The model under review builds one solid part; all positions refer to its coordinate system, in mm. Face numbers are marked on the shaded views. Round coordinates to 2 decimals unless told otherwise and drop trailing zeros. Order: outer loops, then holes, each group sorted by start corner. A loop starts at its lowest first (then second) coordinate and runs counter-clockwise, first axis right, second up.
Autodesk Inventor part; units mm, degrees
ref_plane "YZ Plane" through (0, 0, 0) normal (1, 0, 0) x (0, 1, 0)
ref_plane "XZ Plane" through (0, 0, 0) normal (0, 1, 0) x (-1, 0, 0)
ref_plane "XY Plane" through (0, 0, 0) normal (0, 0, 1) x (1, 0, 0)
sketch "Эскиз1" plane through (0, 0, 0) normal (0, 1, 0) x (-1, 0, 0)
  line L0 (0, 0) -> (2.52, 0)
  line L1 (2.52, 0) -> (2.52, -2.52)
  line L2 (2.52, -2.52) -> (0, -2.52)
  line L3 (0, -2.52) -> (0, 0)
  dimension "d1" = 2.52
  dimension "d2" = 2.52
extrude "Выдавливание1" add sketch "Эскиз1" along normal blind 8
sketch "Эскиз2" plane through (0, 8, 0) normal (0, 1, 0) x (1, 0, 0)
  line L0 (-2.52, 2.52) -> (-2.52, 0) construction
  line L1 (0, 0) -> (0, 2.52) construction
  line L2 (-2.52, 0) -> (0, 2.52) construction
  circle A0 centre (-1.26, 1.26) radius 0.5
  dimension "d22" = 1
extrude "Выдавливание2" add sketch "Эскиз2" along normal blind 3.5
chamfer "Фаска3" distance 0.5 angle 45 1 edges at (-1.76, 11.5, -1.26)
sketch "Эскиз3" plane through (0, 0, 0) normal (0, -1, 0) x (1, 0, 0)
  line L0 (0, 0) -> (0, -2.52) construction
  line L1 (0, -2.52) -> (-2.52, -2.52) construction
  line L2 (0, 0) -> (-2.52, -2.52) construction
  line L3 (-1.81, -0.71) -> (-0.71, -0.71)
  line L4 (-0.71, -0.71) -> (-0.71, -1.81)
  line L5 (-0.71, -1.81) -> (-1.81, -1.81)
  line L6 (-1.81, -1.81) -> (-1.81, -0.71)
  line L7 (-1.81, -0.71) -> (-0.71, -1.81) construction
  line L8 (-0.71, -0.71) -> (-1.81, -1.81) construction
  point P0 (-1.26, -1.26)
  dimension "d15" = 1.1
  dimension "d16" = 1.1
extrude "Выдавливание3" cut sketch "Эскиз3" against normal blind 6
pattern_linear "Прямоуг.массив1" count 6 spacing 2.52 along (0, 0, 1) of "Выдавливание1", "Выдавливание2", "Выдавливание3", "Фаска3"
properties part number "Гребенка 20 МАМА"
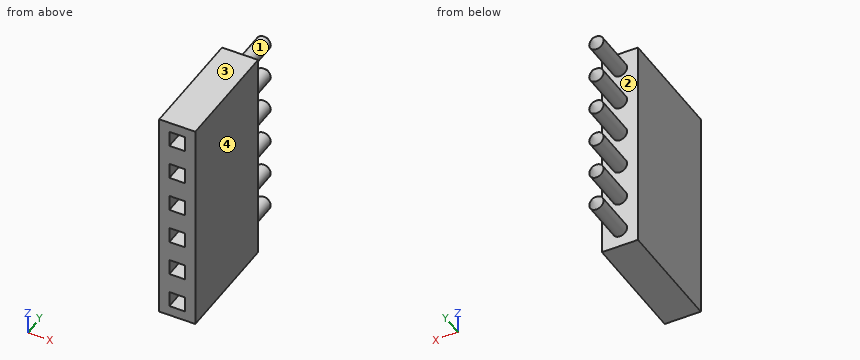
(1) We need section D-D (z = 7.75). Give the boundary of the cut face in (x, y), and give its area (3 significant figures).
(2) To check wall thickness, follow L1, parallel to X at y = 5.5, z = 8.5; L2, parallel to Z at x = -1, y = 8.5; L3, parallel to Y at x = -1, z = 5. State the ranges of each line that lie inside material, in increasing order.
(3) Clearance check with a flat-ended pin moving along its axis: P1, Ø2, axis at y = 9.5, z = 1, coming from the +X side. State where the tip first meets the part, or that it passes through.
(4) We need section A-A (y = 1.5). Give the boundary of the cut face in (x, z).
(5) We need section C-C (x = -2.05). Give the boundary of the cut face in (y, z).
(6) We need section B-B (y = 8.5). Give the boundary of the cut face in (x, z), and give its area (3 significant figures).
(7) The part is to be moulded in two halves that separate along Z. For the marked faces 1, 2, 3 and 4, say which applies: pulls with the +Z half, pulls with the -Z half, needs draft (parallel to the pull), parting line crosses it, or undercut.
Verdict:
1. outline: (-2.52, 0) - (0, 0) - (0, 8) - (-2.52, 8) - close
1. area: 20.2 mm2
2. L1: x = -2.52 to -1.81, -0.71 to 0
2. L2: z = -1.69 to -0.83, 0.83 to 1.69, 3.35 to 4.21, 5.87 to 6.73, 8.39 to 9.25, 10.91 to 11.77
2. L3: y = 0 to 8
3. P1: stops at x = -0.76
4. outline: (-2.52, -2.52) - (0, -2.52) - (0, 12.6) - (-2.52, 12.6) - close; hole (-1.81, -1.81) - (-0.71, -1.81) - (-0.71, -0.71) - (-1.81, -0.71) - close; hole (-1.81, 0.71) - (-0.71, 0.71) - (-0.71, 1.81) - (-1.81, 1.81) - close; hole (-1.81, 3.23) - (-0.71, 3.23) - (-0.71, 4.33) - (-1.81, 4.33) - close; hole (-1.81, 5.75) - (-0.71, 5.75) - (-0.71, 6.85) - (-1.81, 6.85) - close; hole (-1.81, 8.27) - (-0.71, 8.27) - (-0.71, 9.37) - (-1.81, 9.37) - close; hole (-1.81, 10.79) - (-0.71, 10.79) - (-0.71, 11.89) - (-1.81, 11.89) - close
5. outline: (0, -2.52) - (8, -2.52) - (8, 12.6) - (0, 12.6) - close
6. outline: circle Ø1 at (-1.26, -1.26); circle Ø1 at (-1.26, 1.26); circle Ø1 at (-1.26, 3.78); circle Ø1 at (-1.26, 6.3); circle Ø1 at (-1.26, 8.82); circle Ø1 at (-1.26, 11.34)
6. area: 4.71 mm2
7. face 1: undercut
7. face 2: undercut
7. face 3: pulls with the +Z half
7. face 4: needs draft
